```python
from build123d import *

# Parameters (mm, degrees)
SKETCH_2_R          = 1.5
EXTRUDE_1_DEPTH     = 4
CUT_EXTRUDE_1_DEPTH = 2
CHAMFER_1_SIZE      = 0.2
FILLET_1_R          = 0.2


with BuildPart() as part:
    # 草图1 → 旋转1 (revolve)
    with BuildSketch(Plane.XY):
        Polygon((0, 0), (0, -2), (1.5, -2), (3, 0), align=None)
    revolve(axis=Axis((0, 0, 0), (0, -1, 0)))

    # 草图2 → 凸台-拉伸1 (add)
    with BuildSketch(Plane.XZ.offset(2)):
        Circle(SKETCH_2_R)
    extrude(amount=EXTRUDE_1_DEPTH)

    # 草图3 → 切除-拉伸1 (cut)
    with BuildSketch(Plane(origin=(0, 0, 0), x_dir=(1, 0, 0), z_dir=(0, 1, 0))):
        Polygon((-1.327905619, 0), (-0.66395281, -1.15), (0.66395281, -1.15), (1.327905619, 0), (0.66395281, 1.15), (-0.66395281, 1.15), align=None)
    extrude(amount=-CUT_EXTRUDE_1_DEPTH, mode=Mode.SUBTRACT)

    # 倒角1
    chamfer_1_edges = [part.edges().sort_by_distance(p)[0] for p in [
        (-1.5, -6, 0),
    ]]
    chamfer(chamfer_1_edges, length=CHAMFER_1_SIZE)

    # 圆角1
    fillet_1_edges = [part.edges().sort_by_distance(p)[0] for p in [
        (-3, 0, 0),
    ]]
    fillet(fillet_1_edges, radius=FILLET_1_R)


solid = part.part
```
Check sheet for the modelled part. Datum: model origin and axes. Units: mm. A direction names the side the tool comes from. Round coordinates to 2 decimals unless told otherwise and drop trailing zeros. Write each loop counter-clockwise with the first axis right and the second up, starting at its lowest first coordinate (ties: lowest second). Pieces come first, ordered by that corner, then holes. Notation, with made-up numbers: M 0,15 L 47,15 A19 ccw 47,52 Z; hole C 51.25,84 d5. An arc over 180 degrees is marked long. Write item = value, one per line. Start each with the question number.
1. Section check B-B, the plane x = 0. Record the cut outline in (y, z), then the cut area to 3 significant figures.
2. Scan lines: line 1 (Y direction, x = 0.3, z = 1.05); line 2 (Z direction, x = 0, y = -0.25); line 3 (X direction, y = -0.75, z = 0.4). Record each from-to range of solid material in increasing order. Write a range as [from, to].
3. Gauge pin test, flat ends, axial feed: pin 1 (1.5 mm diameter, centred on x = 0, y = -4.5, fed in from -Z); pin 2 (1.5 mm diameter, centred on x = -2, y = -2, fed in from -Z); pin 3 (0.7 mm diameter, centred on x = 0, z = 0, fed in from +Y). Record the tip position at first contact, or that the pin passes through.
4. Tool access check on faces 4 (the flat face through (1, -0.99, -0.57)), 5 (the flat face through (0, -6, 0)). Record the directions out of +Z, -Z, +X, -X, +Y, -Y that give a thin tool (end or side, any length) a straight path to the whole face; none if there is none.
5. Section check C-C, the plane y = -3. Record the cut outline in (x, z), then the cut area to 3 significant figures.
6. Release check for a two-part mould opening along Z. For faces 1 (the flat face through (1, 0, -1)), 2 (the flat face through (0, -1, 1.15)), 3 (the cylindrical face through (-1.5, -3.87, 0.07)) record: pulls with the +Z half, pulls with the -Z half, needs draft (parallel to the pull), parting line crosses it, or undercut.
7. Section check A-A, the plane y = -1. Record the cut outline in (x, z), then the cut area to 3 significant figures.
Results found:
q1.outline = M -6,-1.3 L -5.8,-1.5 L -2,-1.5 L -0.32,-2.76 A0.2 ccw 0,-2.6 L 0,-1.15 L -2,-1.15 L -2,1.15 L 0,1.15 L 0,2.6 A0.2 ccw -0.32,2.76 L -2,1.5 L -5.8,1.5 L -6,1.3 Z
q1.area = 16.3 mm^2
q2.line_1 = [-6, -2]
q2.line_2 = [-2.79, -1.15], [1.15, 2.79]
q2.line_3 = [-2.4, -1.1], [1.1, 2.4]
q3.pin_1 = -1.5
q3.pin_2 = -1.2
q3.pin_3 = -2
q4.face_4 = +Y
q4.face_5 = +Z, -Z, +X, -X, -Y
q5.outline = C 0,0 d3
q5.area = 7.07 mm^2
q6.face_1 = needs draft
q6.face_2 = undercut
q6.face_3 = parting line crosses it
q7.outline = C 0,0 d4.5; hole M -1.33,0 L -0.66,-1.15 L 0.66,-1.15 L 1.33,0 L 0.66,1.15 L -0.66,1.15 Z
q7.area = 11.3 mm^2
